from build123d import *

# Parameters (mm, degrees)
SKETCH1_W           = 115
SKETCH1_H           = 102
BOSS_EXTRUDE1_DEPTH = 4
SKETCH3_W           = 15
SKETCH3_H           = 90
BOSS_EXTRUDE2_DEPTH = 40
SKETCH4_R           = 2.125
CUT_EXTRUDE4_DEPTH  = 10
SKETCH11_W          = 104
SKETCH11_H          = 91
CUT_EXTRUDE5_DEPTH  = 2
SKETCH14_R          = 1
CUT_EXTRUDE7_DEPTH  = 20
BOSS_EXTRUDE4_DEPTH = 70
SKETCH13_R          = 1
CUT_EXTRUDE6_DEPTH  = 20
SKETCH7_W           = 115
SKETCH7_H           = 102
BOSS_EXTRUDE5_DEPTH = 4
SKETCH8_R           = 2
CUT_EXTRUDE2_DEPTH  = 2
SKETCH9_R           = 1.5
CUT_EXTRUDE3_DEPTH  = 2
SKETCH15_W          = 168.231856539
SKETCH15_H          = 129.587124708
CUT_EXTRUDE8_DEPTH  = 171.601875722


with BuildPart() as part:
    # Sketch1 → Boss-Extrude1 (new body)
    with BuildSketch(Plane(origin=(0, 0, 0), x_dir=(1, 0, 0), z_dir=(0, 1, 0))):
        with Locations((57.5, 51)):
            Rectangle(SKETCH1_W, SKETCH1_H)
    extrude(amount=BOSS_EXTRUDE1_DEPTH)

    # Sketch3 → Boss-Extrude2 (add)
    with BuildSketch(Plane.XZ):
        with Locations((13, -51)):
            Rectangle(SKETCH3_W, SKETCH3_H)
        with Locations((102, -51)):
            Rectangle(SKETCH3_W, SKETCH3_H)
    extrude(amount=BOSS_EXTRUDE2_DEPTH)

    # Sketch4 → Cut-Extrude4 (cut)
    with BuildSketch(Plane.XZ.offset(40)):
        with Locations(Location((14.525, -67.125, 0), (0, 0, 270))):
            Circle(SKETCH4_R)
        with Locations(Location((14.525, -34.875, 0), (0, 0, 270))):
            Circle(SKETCH4_R)
        with Locations(Location((100.475, -67.125, 0), (0, 0, 270))):
            Circle(SKETCH4_R)
        with Locations(Location((100.475, -34.875, 0), (0, 0, 270))):
            Circle(SKETCH4_R)
    extrude(amount=-CUT_EXTRUDE4_DEPTH, mode=Mode.SUBTRACT)

    # Sketch11 → Cut-Extrude5 (cut)
    with BuildSketch(Plane(origin=(0, 4, 0), x_dir=(1, 0, 0), z_dir=(0, 1, 0))):
        with Locations((57.5, 51)):
            Rectangle(SKETCH11_W, SKETCH11_H)
    extrude(amount=-CUT_EXTRUDE5_DEPTH, mode=Mode.SUBTRACT)

    # Sketch14 → Cut-Extrude7 (cut)
    with BuildSketch(Plane.XZ):
        with Locations(Location((109, -100, 0), (0, 0, 270))):
            Circle(SKETCH14_R)
        with Locations(Location((113, -96, 0), (0, 0, 270))):
            Circle(SKETCH14_R)
        with Locations(Location((2, -96, 0), (0, 0, 270))):
            Circle(SKETCH14_R)
        with Locations(Location((6, -100, 0), (0, 0, 270))):
            Circle(SKETCH14_R)
        with Locations(Location((113, -6, 0), (0, 0, 270))):
            Circle(SKETCH14_R)
        with Locations(Location((109, -2, 0), (0, 0, 270))):
            Circle(SKETCH14_R)
        with Locations(Location((2, -6, 0), (0, 0, 270))):
            Circle(SKETCH14_R)
        with Locations(Location((6, -2, 0), (0, 0, 270))):
            Circle(SKETCH14_R)
    extrude(amount=-CUT_EXTRUDE7_DEPTH, mode=Mode.SUBTRACT)

    # Sketch6 → Boss-Extrude4 (add)
    with BuildSketch(Plane(origin=(0, 4, 0), x_dir=(1, 0, 0), z_dir=(0, 1, 0))):
        Polygon((0, 0), (0, 8), (4, 8), (4, 4), (8, 4), (8, 0), align=None)
        Polygon((107, 0), (115, 0), (115, 8), (111, 8), (111, 4), (107, 4), align=None)
        Polygon((107, 102), (115, 102), (115, 94), (111, 94), (111, 98), (107, 98), align=None)
        Polygon((8, 102), (0, 102), (0, 94), (4, 94), (4, 98), (8, 98), align=None)
    extrude(amount=BOSS_EXTRUDE4_DEPTH)

    # Sketch13 → Cut-Extrude6 (cut)
    with BuildSketch(Plane.XZ):
        with Locations(Location((109, -100, 0), (0, 0, 270))):
            Circle(SKETCH13_R)
        with Locations(Location((113, -96, 0), (0, 0, 270))):
            Circle(SKETCH13_R)
        with Locations(Location((2, -96, 0), (0, 0, 90))):
            Circle(SKETCH13_R)
        with Locations(Location((6, -100, 0), (0, 0, 90))):
            Circle(SKETCH13_R)
        with Locations(Location((113, -6, 0), (0, 0, 90))):
            Circle(SKETCH13_R)
        with Locations(Location((109, -2, 0), (0, 0, 90))):
            Circle(SKETCH13_R)
        with Locations(Location((6, -2, 0), (0, 0, 270))):
            Circle(SKETCH13_R)
        with Locations(Location((2, -6, 0), (0, 0, 270))):
            Circle(SKETCH13_R)
    extrude(amount=-CUT_EXTRUDE6_DEPTH, mode=Mode.SUBTRACT)

    # Sketch7 → Boss-Extrude5 (add)
    with BuildSketch(Plane(origin=(0, 74, 0), x_dir=(1, 0, 0), z_dir=(0, 1, 0))):
        with Locations((57.5, 51)):
            Rectangle(SKETCH7_W, SKETCH7_H)
    extrude(amount=BOSS_EXTRUDE5_DEPTH)

    # Sketch8 → Cut-Extrude2 (cut)
    with BuildSketch(Plane(origin=(0, 78, 0), x_dir=(1, 0, 0), z_dir=(0, 1, 0))):
        with Locations(Location((29.25, 79, 0), (0, 0, 270))):
            Circle(SKETCH8_R)
        with Locations(Location((85.25, 79, 0), (0, 0, 270))):
            Circle(SKETCH8_R)
        with Locations(Location((37.5, 9, 0), (0, 0, 270))):
            Circle(SKETCH8_R)
        with Locations(Location((77.5, 9, 0), (0, 0, 270))):
            Circle(SKETCH8_R)
    extrude(amount=-CUT_EXTRUDE2_DEPTH, mode=Mode.SUBTRACT)

    # Sketch9 → Cut-Extrude3 (cut)
    with BuildSketch(Plane(origin=(0, 78, 0), x_dir=(1, 0, 0), z_dir=(0, 1, 0))):
        with Locations(Location((52.1, 90.9, 0), (0, 0, 270))):
            Circle(SKETCH9_R)
        with Locations(Location((85.6, 14.4, 0), (0, 0, 270))):
            Circle(SKETCH9_R)
        with Locations(Location((29.8, 11.3, 0), (0, 0, 270))):
            Circle(SKETCH9_R)
    extrude(amount=-CUT_EXTRUDE3_DEPTH, mode=Mode.SUBTRACT)

    # Sketch15 → Cut-Extrude8 (cut, through all)
    with BuildSketch(Plane(origin=(0, 4, 0), x_dir=(1, 0, 0), z_dir=(0, 1, 0))):
        with Locations((71.077613374, 52.272730689)):
            Rectangle(SKETCH15_W, SKETCH15_H)
    extrude(amount=-CUT_EXTRUDE8_DEPTH, mode=Mode.SUBTRACT)


solid = part.part
Build history of the part. All positions in model axes, mm. A direction names the side the tool comes from. Give positions to 0.01 mm unless a question says otherwise; leave off trailing zeros. Order: outer loops, then holes, each group sorted by start corner. A loop starts at its lowest first (then second) coordinate and runs counter-clockwise, first axis right, second up. Notation, with made-up numbers: M 56,-38.75 L 107,-38.75 A14 cw 107,-34.75 Z; hole C 77.25,88 d11. An arc over 180 degrees is marked long. Use one line per item in the form item = value.
Q1. Which spindle directions (+Z, -Z, +X, -X, +Y, -Y) get a long thin tool onto all of the face, cutting with end or side? Do faces 1 (the flat face through (6, 39, -4)), 2 (the flat face through (107, 39, -2)), 3 (the flat face through (113, 39, -94)), 4 (the flat face through (29, 76, -79)). Say none if no direction does.
Conclusion:
face_1 = -Y
face_2 = +Z, -Z, -Y
face_3 = +X, -X, -Y
face_4 = +Y
Q2. Slice it at A-A, the plane y = 44.5. Write the cut outline in (x, z), and give its area (3 significant figures).
Conclusion:
outline = M 0,-102 L 8,-102 L 8,-98 L 4,-98 L 4,-94 L 0,-94 Z; M 0,-8 L 4,-8 L 4,-4 L 8,-4 L 8,0 L 0,0 Z; M 107,-102 L 115,-102 L 115,-94 L 111,-94 L 111,-98 L 107,-98 Z; M 107,-4 L 111,-4 L 111,-8 L 115,-8 L 115,0 L 107,0 Z
area = 192 mm2
Q3. Pin check, flat tips, straight feed: P1, Ø12, axis at y = 67, z = -55.5, coming from the -X side; P2, Ø10, axis at x = 72.5, z = -11.5, coming from the -Y side; P3, Ø0.6, axis at x = 113, z = -96, coming from the -Y side; P4, Ø2, axis at x = 37.5, z = -9, coming from the +Y side. Stop position of each tip, or through.
Conclusion:
P1 = through
P2 = 74
P3 = 20
P4 = 76
Q4. Pull direction Z, two halves, no side cores. Call faces 5 (the flat face through (107, 39, -100)), 6 (the flat face through (4, 39, -96)): released by +Z, released by -Z, zero draft, split by the parting line, or undercut.
Conclusion:
face_5 = zero draft
face_6 = undercut
Q5. Slice it at D-D, the plane z = -79. Write the cut outline in (x, y).
Conclusion:
outline = M 0,74 L 115,74 L 115,78 L 87.25,78 L 87.25,76 L 83.25,76 L 83.25,78 L 31.25,78 L 31.25,76 L 27.25,76 L 27.25,78 L 0,78 Z
Q6. Slice it at C-C, the plane x = 37.5. Write the cut outline in (y, z), and give its area (3 significant figures).
Conclusion:
outline = M 74,-102 L 78,-102 L 78,-11 L 76,-11 L 76,-7 L 78,-7 L 78,0 L 74,0 Z
area = 400 mm2
Q7. Slice it at B-B, the plane z = -14.4. Write the cut outline in (x, y).
Conclusion:
outline = M 0,74 L 115,74 L 115,78 L 87.1,78 L 87.1,76 L 84.1,76 L 84.1,78 L 0,78 Z
Q8. Wall check: probe 1 along X at (y, z) = (10, -100); probe 2 along Z at (x, y) = (85.6, 77.25); probe 3 along X at (y, z) = (14.75, -96). Give the ranges that are in metal, low to high.
Conclusion:
probe_1 = 0 to 5, 7 to 8, 107 to 108, 110 to 115
probe_2 = -102 to -80.97, -77.03 to -15.9, -12.9 to 0
probe_3 = 0 to 1, 3 to 4, 111 to 112, 114 to 115
